from build123d import *

# Parameters (mm, degrees)
SKETCH1_R           = 1.5
SKETCH1_R_2         = 4
BOSS_EXTRUDE1_DEPTH = 2
SKETCH5_R           = 1.5
SKETCH5_R_2         = 4
BOSS_EXTRUDE4_DEPTH = 2
SKETCH6_W           = 25
SKETCH6_H           = 56
BOSS_EXTRUDE5_DEPTH = 2
FILLET2_R           = 1
SKETCH7_R           = 4
SKETCH7_R_2         = 1.5
CUT_EXTRUDE1_DEPTH  = 2


with BuildPart() as part:
    # Sketch1 → Boss-Extrude1 (new body)
    with BuildSketch(Plane.XY):
        with BuildLine():
            Line((-12.5, -32.5), (12.5, -32.5))
            Line((12.5, -32.5), (12.5, 7.5))
            Line((12.5, 7.5), (12.5, 20))
            ThreePointArc((12.5, 20), (8.838834758, 28.838834772), (-2e-08, 32.5))
            ThreePointArc((-2e-08, 32.5), (-8.838834772, 28.838834758), (-12.5, 20))
            Line((-12.5, 20), (-12.5, 7.5))
            Line((-12.5, 7.5), (-12.5, -32.5))
        make_face()
        with Locations((0, -17.5)):
            Circle(SKETCH1_R, mode=Mode.SUBTRACT)
        Circle(SKETCH1_R, mode=Mode.SUBTRACT)
        with Locations((0, 12.5)):
            Circle(SKETCH1_R, mode=Mode.SUBTRACT)
        with Locations((-7.5, 20)):
            Circle(SKETCH1_R, mode=Mode.SUBTRACT)
        with Locations((0, 20)):
            Circle(SKETCH1_R_2, mode=Mode.SUBTRACT)
        with Locations((0, 27.5)):
            Circle(SKETCH1_R, mode=Mode.SUBTRACT)
        with Locations((7.5, 20)):
            Circle(SKETCH1_R, mode=Mode.SUBTRACT)
    extrude(amount=BOSS_EXTRUDE1_DEPTH)



with BuildPart() as body_2:
    # Sketch5 → Boss-Extrude4 (new body)
    with BuildSketch(Plane.XY.offset(54)):
        with BuildLine():
            Line((-12.5, -32.5), (12.5, -32.5))
            Line((12.5, -32.5), (12.5, 7.5))
            Line((12.5, 7.5), (12.5, 20))
            ThreePointArc((12.5, 20), (8.838834758, 28.838834772), (-2e-08, 32.5))
            ThreePointArc((-2e-08, 32.5), (-8.838834772, 28.838834758), (-12.5, 20))
            Line((-12.5, 20), (-12.5, 7.5))
            Line((-12.5, 7.5), (-12.5, -32.5))
        make_face()
        with Locations((0, -17.5)):
            Circle(SKETCH5_R, mode=Mode.SUBTRACT)
        Circle(SKETCH5_R, mode=Mode.SUBTRACT)
        with Locations((0, 12.5)):
            Circle(SKETCH5_R, mode=Mode.SUBTRACT)
        with Locations((-7.5, 20)):
            Circle(SKETCH5_R, mode=Mode.SUBTRACT)
        with Locations((0, 20)):
            Circle(SKETCH5_R_2, mode=Mode.SUBTRACT)
        with Locations((0, 27.5)):
            Circle(SKETCH5_R, mode=Mode.SUBTRACT)
        with Locations((7.5, 20)):
            Circle(SKETCH5_R, mode=Mode.SUBTRACT)
    extrude(amount=BOSS_EXTRUDE4_DEPTH)


with BuildPart() as part_1:
    add(part.part)

    add(body_2.part)  # Boss-Extrude5 merges body 2
    # Sketch6 → Boss-Extrude5 (add)
    with BuildSketch(Plane.XZ.offset(32.5)):
        with Locations((0, 28)):
            Rectangle(SKETCH6_W, SKETCH6_H)
    extrude(amount=-BOSS_EXTRUDE5_DEPTH)

    # Fillet2
    fillet2_edges = [part_1.edges().sort_by_distance(p)[0] for p in [
        (0, -32.5, 0),
        (0, -32.5, 56),
    ]]
    fillet(fillet2_edges, radius=FILLET2_R)

    # Sketch7 → Cut-Extrude1 (cut)
    with BuildSketch(Plane(origin=(0, -32.5, 0), x_dir=(-1, 0, 0), z_dir=(0, -1, 0))):
        with Locations(Location((0, -28, 0), (0, 0, 90))):
            Circle(SKETCH7_R)
        with Locations(Location((7.5, -28, 0), (0, 0, 90))):
            Circle(SKETCH7_R_2)
        with Locations(Location((0, -35.5, 0), (0, 0, 90))):
            Circle(SKETCH7_R_2)
        with Locations(Location((-7.5, -28, 0), (0, 0, 90))):
            Circle(SKETCH7_R_2)
        with Locations(Location((0, -20.5, 0), (0, 0, 90))):
            Circle(SKETCH7_R_2)
        with Locations(Location((0, -46.5, 0), (0, 0, 90))):
            Circle(SKETCH7_R_2)
        with Locations(Location((0, -9.5, 0), (0, 0, 90))):
            Circle(SKETCH7_R_2)
    extrude(amount=-CUT_EXTRUDE1_DEPTH, mode=Mode.SUBTRACT)


solid = part_1.part
Input: part model. Units: mm. Frame: model coordinates. Round coordinates to 2 decimals unless told otherwise and drop trailing zeros. Loops run counter-clockwise (first coordinate to the right, second up) from the corner with the lowest first, then second, coordinate; pieces in that order, holes last. Notation, with made-up numbers: (21, 8) -> (70, 8) arc R21 cw to (70, 37) -> close; hole circle Ø9 at (-6.75, 78.5). An arc over 180 degrees is marked (long way). Answer as a JSON object with one key per item and string values. Group by question number.
1) Pin query (flat end, axial travel): pin 1 (6 mm diameter, centred on x = -9, z = 19, fed in from +Y); pin 2 (12 mm diameter, centred on x = -1, y = 16.5, fed in from -Z). Return the tip coordinate at first contact, or that it passes through.
2) Section query C-C on z = 9.5. Output: boundary loops of the cut face in (x, y), plus the area to 3 significant figures.
3) Section query A-A on y = -17.5. Output: boundary loops of the cut face in (x, z), plus the area to 3 significant figures.
4) Section query D-D on y = 27.5. Output: boundary loops of the cut face in (x, z), plus the area to 3 significant figures.
5) Draft query along Z for faces 1 (the cylindrical face through (0, -16, 1)), 2 (the flat face through (3, 1, 56)), 3 (the flat face through (3, 1, 54)). Return one class per face: +Z half, -Z half, draft (parallel to the pull), parting line (faces both ways), or undercut.
6) Ray query, L1, parallel to Y at x = 0, z = 1.6; L2, parallel to Z at x = 2.25, y = 1; L3, parallel to Y at x = -2.75, z = 4.5. Return the intervals inside material, ascending.
7) Section query B-B on x = -7.5. Output: boundary loops of the cut face in (y, z).
Reply:
{
 "1": {"pin 1": "stops at y = -30.5", "pin 2": "stops at z = 0"},
 "2": {"outline": "(-12.5, -32.5) -> (-1.5, -32.5) -> (-1.5, -30.5) -> (-12.5, -30.5) -> close; (1.5, -32.5) -> (12.5, -32.5) -> (12.5, -30.5) -> (1.5, -30.5) -> close", "area": "44.0 mm2"},
 "3": {"outline": "(-12.5, 0) -> (-1.5, 0) -> (-1.5, 2) -> (-12.5, 2) -> close; (-12.5, 54) -> (-1.5, 54) -> (-1.5, 56) -> (-12.5, 56) -> close; (1.5, 0) -> (12.5, 0) -> (12.5, 2) -> (1.5, 2) -> close; (1.5, 54) -> (12.5, 54) -> (12.5, 56) -> (1.5, 56) -> close", "area": "88.0 mm2"},
 "4": {"outline": "(-10, 0) -> (-1.5, 0) -> (-1.5, 2) -> (-10, 2) -> close; (-10, 54) -> (-1.5, 54) -> (-1.5, 56) -> (-10, 56) -> close; (1.5, 0) -> (10, 0) -> (10, 2) -> (1.5, 2) -> close; (1.5, 54) -> (10, 54) -> (10, 56) -> (1.5, 56) -> close", "area": "68.0 mm2"},
 "5": {"face 1": "draft", "face 2": "+Z half", "face 3": "undercut"},
 "6": {"L1": "y = -32.5 to -19, -16 to -1.5, 1.5 to 11, 14 to 16, 24 to 26, 29 to 32.5", "L2": "z = 0 to 2, 54 to 56", "L3": "y = -32.5 to -30.5"},
 "7": {"outline": "(-32.5, 1) arc R1 ccw to (-31.5, 0) -> (18.5, 0) -> (18.5, 2) -> (-30.5, 2) -> (-30.5, 26.5) -> (-32.5, 26.5) -> close; (-32.5, 29.5) -> (-30.5, 29.5) -> (-30.5, 54) -> (18.5, 54) -> (18.5, 56) -> (-31.5, 56) arc R1 ccw to (-32.5, 55) -> close; (21.5, 0) -> (30, 0) -> (30, 2) -> (21.5, 2) -> close; (21.5, 54) -> (30, 54) -> (30, 56) -> (21.5, 56) -> close"}
}
